Read the model definition and answer for the solid it produces. Units are mm, in the model's axes. A direction names the side the tool comes from. Coordinates: 2 decimals unless noted, no trailing zeros. Loops run counter-clockwise (first coordinate to the right, second up) from the corner with the lowest first, then second, coordinate; pieces in that order, holes last. Notation, with made-up numbers: M 50.25,-11.5 L 106.25,-11.5 A24 ccw 106.25,26.5 Z; hole C -36.75,2.5 d4. An arc over 180 degrees is marked long. One line per item, written item: value. Start each with the question number.
```python
from build123d import *

# Parameters (mm, degrees)
F1_DEPTH    = 2.75
F2_T1_DEPTH = 30.499500005
F3_R        = 10
F6_DEPTH    = 31.7539349198
F7_R        = 15
F8_R        = 10


# Not quite as in the source:
# - a fillet or chamfer that OpenCascade refuses, or shapes differently, is made with other operations: its cross-section is extruded or revolved along the edge and cut away or added


with BuildPart() as f1:
    # F0 (on Front) → F1 (new body, symmetric)
    with BuildSketch(Plane.XZ):
        Polygon((0, 230), (0, 0), (31.8198051534, -31.8198051534), (40.3050865276, -23.3345237792), (5.5, 11.4705627485), (5.5, 230), align=None)
    extrude(amount=F1_DEPTH, both=True)

    # F2: fillet of radius 5 on 2 edges, made by hand

    # F2_s2 → F2_t1 (cut)
    with BuildSketch(Plane.XZ.offset(-15.2497500025)):
        with BuildLine():
            ThreePointArc((35.3553390593, -28.2844126688), (31.8198051534, -29.7488787629), (28.2842712475, -28.2844126688))
            Line((28.2842712475, -28.2844126688), (28.2135605693, -28.3551233469))
            ThreePointArc((28.2135605693, -28.3551233469), (29.9813628776, -30.1227842339), (31.7490944753, -31.8905158315))
            Line((31.7490944753, -31.8905158315), (31.8905158315, -31.8905158315))
            ThreePointArc((31.8905158315, -31.8905158315), (33.6582474291, -30.1227842339), (35.4260497374, -28.3551233469))
            Line((35.4260497374, -28.3551233469), (35.3553390593, -28.2844126688))
        make_face()
        with BuildLine():
            ThreePointArc((36.7696940431, -19.7989898732), (38.2341601371, -23.3345237792), (36.7696940431, -26.8700576851))
            Line((36.7696940431, -26.8700576851), (36.8404047212, -26.9407683632))
            ThreePointArc((36.8404047212, -26.9407683632), (38.6080656081, -25.1729660549), (40.3757972058, -23.4052344573))
            Line((40.3757972058, -23.4052344573), (40.3757972058, -23.263813101))
            ThreePointArc((40.3757972058, -23.263813101), (38.6080656081, -21.4960815034), (36.8404047212, -19.7282791951))
            Line((36.8404047212, -19.7282791951), (36.7696940431, -19.7989898732))
        make_face()
    extrude(amount=F2_T1_DEPTH, mode=Mode.SUBTRACT)

    # F3
    f3_edges = [f1.edges().sort_by_distance(p)[0] for p in [
        (0, 0, 0),
    ]]
    fillet(f3_edges, radius=F3_R)

    # F5 (on offset) → F6 (cut)
    with BuildSketch(Plane(origin=(0, 0, 0), x_dir=(0.7071067812, 0, -0.7071067812), z_dir=(-0.7071067812, 0, -0.7071067812))):
        Polygon((40, 2.75), (-8.2739908248, 2.75), (0.2329319046, 1.25), (45, 1.25), (45, 2.75), align=None)
    extrude(amount=-F6_DEPTH, mode=Mode.SUBTRACT)

    # F7
    f7_edges = [f1.edges().sort_by_distance(p)[0] for p in [
        (5.5, 0.357253, 11.470563),
    ]]
    fillet(f7_edges, radius=F7_R)

    # F8
    f8_edges = [f1.edges().sort_by_distance(p)[0] for p in [
        (2.753762, -2.75, 14.454952),
        (4.725257, -1.25, 4.395842),
    ]]
    fillet(f8_edges, radius=F8_R)


solid = f1.part
```
1) Consider line 1 along X through (y, z) = (1.7, 61.5); line 2 along Z through (x, y) = (15.5, -0.3); line 3 along Z through (x, y) = (25, -0.6). Determine where each line is inside the solid, lowest interval first.
2) Section C-C (x = 23.5) is taken. Determine the outline of the cut face in (y, z).
3) Section A-A (y = 1.9) is taken. Determine the outline of the cut face in (x, z), then the cut area to 3 significant figures.
4) Section B-B (z = 148) is taken. Determine the outline of the cut face in (x, y), then the cut area to 4 significant figures.
5) A tool of negligible diameter and unlimited length cuts with its end or side. For faces 1 (the face through (5.5, 0, 122)), 2 (the face through (15, 1, -15)), from which of +Z, -Z, +X, -X, +Y, -Y can it reach the whole face along a straight path? Write none if from no direction.
6) A flat-ended cylindrical pin translates along its axis: pin 1 (1.5 mm diameter, centred on x = 16, y = -1.5, fed in from +Z). Find the tip coordinate at first contact, or state that the pin passes through.
Results found:
1. line 1: x = 0 to 5.5
1. line 2: z = -15.5 to 1.47
1. line 3: z = -25 to -8.03
2. outline: M -1.25,-23.5 L 2.75,-23.5 L 2.75,-6.53 L -1.25,-6.53 Z
3. outline: M 0,4.14 A10 ccw 2.93,-2.93 L 28.31,-28.31 A5 ccw 35.33,-28.31 L 36.79,-26.85 A5 ccw 36.79,-19.82 L 9.89,7.08 A15 cw 5.5,17.68 L 5.5,230 L 0,230 Z
3. area: 1,790 mm²
4. outline: M 0,-2.75 L 5.5,-2.75 L 5.5,2.75 L 0,2.75 Z
4. area: 30.25 mm²
5. face 1: +Z, +X, +Y, -Y
5. face 2: -Z, -X, +Y, -Y
6. pin 1: stops at z = 1.68
